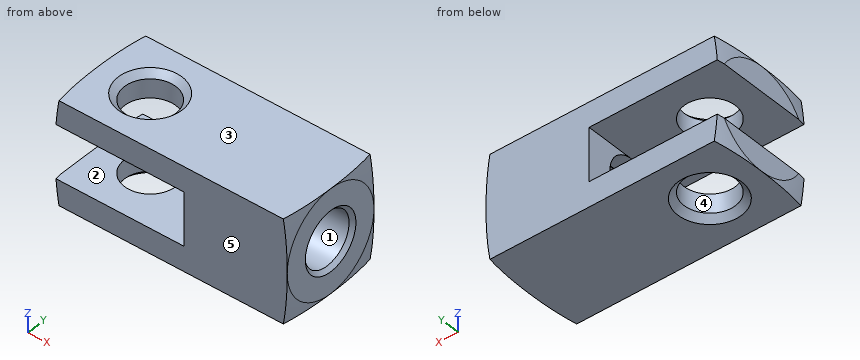
from build123d import *

# Parameters (mm, degrees)
SKETCH1_W                = 42.8752
SKETCH1_H                = 19.05
BOSS_EXTRUDE1_DEPTH      = 9.525
BOSS_EXTRUDE1_DEPTH_BACK = 9.525
SKETCH2_W                = 23.8252
SKETCH2_H                = 9.8425
CUT_EXTRUDE1_DEPTH       = 9.525
CUT_EXTRUDE1_DEPTH_BACK  = 9.525
HOLE1_D                  = 9.73836
HOLE1_DEPTH              = 15.748
HOLE1_CSINK_D            = 11.1125
HOLE1_CSINK_ANGLE        = 90
SKETCH5_W                = 4.96062
SKETCH5_H                = 3.302


with BuildPart() as part:
    # Sketch1 → Boss-Extrude1 (new body, two sides)
    with BuildSketch(Plane.XY) as boss_extrude1_sk:
        with Locations((11.8872, 0)):
            Rectangle(SKETCH1_W, SKETCH1_H)
    extrude(amount=BOSS_EXTRUDE1_DEPTH)
    extrude(boss_extrude1_sk.sketch, amount=-BOSS_EXTRUDE1_DEPTH_BACK)

    # Sketch2 → Cut-Extrude1 (cut, two sides)
    with BuildSketch(Plane(origin=(0, 0, 0), x_dir=(1, 0, 0), z_dir=(0, 1, 0))) as cut_extrude1_sk:
        with Locations((2.3622, 0)):
            Rectangle(SKETCH2_W, SKETCH2_H)
    extrude(amount=CUT_EXTRUDE1_DEPTH, mode=Mode.SUBTRACT)
    extrude(cut_extrude1_sk.sketch, amount=-CUT_EXTRUDE1_DEPTH_BACK, mode=Mode.SUBTRACT)

    # Hole1
    with Locations(Plane(origin=(33.3248, 0, 0), x_dir=(0, 0, -1), z_dir=(1, 0, 0))):
        with Locations((0, 0)):
            CounterSinkHole(HOLE1_D / 2, HOLE1_CSINK_D / 2, depth=HOLE1_DEPTH, counter_sink_angle=HOLE1_CSINK_ANGLE)

    # Sketch5 → Hole2 (revolve, cut)
    with BuildSketch(Plane(origin=(17.5768, 0, 0), x_dir=(0, 0, -1), z_dir=(0, 1, 0))):
        with Locations((2.48031, 1.651)):
            Rectangle(SKETCH5_W, SKETCH5_H)
    revolve(axis=Axis((-92.4232, 0, 0), (1, 0, 0)), mode=Mode.SUBTRACT)

    # Sketch7 → Cut-Revolve1 (revolve, cut)
    with BuildSketch(Plane(origin=(0, 0, 0), x_dir=(0, 0, -1), z_dir=(1, 0, 0))):
        Polygon((-9.525, 0), (-9.525, 5.8674), (-8.382, 4.7244), (8.382, 4.7244), (9.525, 5.8674), (9.525, 0), align=None)
    revolve(axis=Axis((0, 0, -9.525), (0, 0, 1)), mode=Mode.SUBTRACT)

    # Sketch8 → Cut-Revolve2 (revolve, cut)
    with BuildSketch(Plane.XY):
        with BuildLine():
            Line((33.3248, 0), (33.3248, 9.525))
            ThreePointArc((33.3248, 9.525), (32.370901294, 14.371793679), (30.7848, 19.05))
            Line((30.7848, 19.05), (42.8498, 19.05))
            Line((42.8498, 19.05), (42.8498, 0))
            Line((42.8498, 0), (33.3248, 0))
        make_face()
    revolve(axis=Axis((42.8498, 0, 0), (-1, 0, 0)), mode=Mode.SUBTRACT)

    # Sketch9 → Cut-Revolve3 (revolve, cut)
    with BuildSketch(Plane.XY):
        with BuildLine():
            Line((-19.0754, 0), (-19.0754, 19.05))
            Line((-19.0754, 19.05), (-7.0104, 19.05))
            ThreePointArc((-7.0104, 19.05), (-8.596501294, 14.371793679), (-9.5504, 9.525))
            Line((-9.5504, 9.525), (-9.5504, 0))
            Line((-9.5504, 0), (-19.0754, 0))
        make_face()
    revolve(axis=Axis((-9.5504, 0, 0), (-1, 0, 0)), mode=Mode.SUBTRACT)


solid = part.part
Here's how the part is built. I have some questions about the finished solid (model axes, mm). Face numbers are marked on the shaded views. A direction names the side the tool comes from. Round coordinates to 2 decimals unless told otherwise and drop trailing zeros. Loops run counter-clockwise (first coordinate to the right, second up) from the corner with the lowest first, then second, coordinate; pieces in that order, holes last. Notation, with made-up numbers: (25, 19.25) - (44, 19.25) arc R17 cw to (44, 48.25) - close; hole circle Ø1 at (37.25, 47). An arc over 180 degrees is marked (long way). One line per question, with ' | ' between items. Start each with the question number.
Q1. We'd pull the mould along Y, two halves only. Please class the marked faces 3, 4 and 5: +Y half, -Y half, draft (parallel to the pull), parting line (faces both ways), or undercut.
Q2. For the marked faces 1 and 2, which set-ups out of +Z, -Z, +X, -X, +Y, -Y let a thin tool reach every point of the face, with its end or its side?
Q3. Please list where these lines run through material, in increasing order: line 1 (Z direction, x = 15.05, y = 0) (3 decimals); line 2 (Z direction, x = 29.75, y = 0) (3 decimals); line 3 (Y direction, x = 0, z = -6.5) (3 decimals). Write a range as [from, to].
Q4. I want a section at C-C (y = -1.5). State how many separate pieces and enclosed holes the cut face has, then the cut area to 3 significant figures.
Q5. I want a section at B-B (x = 0). Write out the boundary of the cut face in (y, z) (3 decimals), then the cut area to 3 significant figures.
Q6. Will these pins go through, and if not, where does the flat tip stop? pin 1 (7.5 mm diameter, centred on x = 0, y = 0, fed in from +Z); pin 2 (2 mm diameter, centred on y = -4, z = 0.5, fed in from +X); pin 3 (4.5 mm diameter, centred on y = -6, z = -1.5, fed in from -X).
Q7. I want a section at A-A (x = 7). Write out the boundary of the cut face in (y, z) (3 decimals), then the cut area to 3 significant figures.
Response values:
1) face 3: draft | face 4: undercut | face 5: -Y half
2) face 1: +X, -X | face 2: -X, +Y, -Y
3) line 1: z = [-9.525, -4.961], [4.961, 9.525] | line 2: z = [-9.525, -4.869], [4.869, 9.525] | line 3: y = [-9.525, -4.724], [4.724, 9.525]
4) separate pieces: 4 | enclosed holes: 0 | area: 319 mm²
5) outline: (-9.525, -9.525) - (-5.867, -9.525) - (-4.724, -8.382) - (-4.724, -4.921) - (-9.525, -4.921) - close; (-9.525, 4.921) - (-4.724, 4.921) - (-4.724, 8.382) - (-5.867, 9.525) - (-9.525, 9.525) - close; (4.724, -8.382) - (5.867, -9.525) - (9.525, -9.525) - (9.525, -4.921) - (4.724, -4.921) - close; (4.724, 4.921) - (9.525, 4.921) - (9.525, 9.525) - (5.867, 9.525) - (4.724, 8.382) - close | area: 85.8 mm²
6) pin 1: passes through | pin 2: stops at x = 32.8 | pin 3: stops at x = 14.27
7) outline: (-9.525, -9.525) - (9.525, -9.525) - (9.525, -4.921) - (-9.525, -4.921) - close; (-9.525, 4.921) - (9.525, 4.921) - (9.525, 9.525) - (-9.525, 9.525) - close | area: 175 mm²
